Geometry: final body of the model. Coordinates: model frame, mm. A direction names the side the tool comes from. Give positions to 0.01 mm unless a question says otherwise; leave off trailing zeros. Order: outer loops, then holes, each group sorted by start corner. A loop starts at its lowest first (then second) coordinate and runs counter-clockwise, first axis right, second up. Notation, with made-up numbers: (85.25, -38.75) - (105.25, -38.75) arc R19 cw to (105.25, -21.75) - close; hole circle Ø7 at (2.5, -38). An arc over 180 degrees is marked (long way). One line per item, written item: value.
```python
from build123d import *

# Parameters (mm, degrees)
SKETCH1_R           = 1.651
SKETCH1_R_2         = 1.2446
BOSS_EXTRUDE1_DEPTH = 5.08
SKETCH2_R           = 5.40385
SKETCH2_R_2         = 4.1656
BOSS_EXTRUDE2_DEPTH = 1.0922
CHAMFER1_SIZE       = 0.889
SKETCH4_R           = 5.4102
SKETCH4_R_2         = 4.1656
BOSS_EXTRUDE3_DEPTH = 1.4986
CHAMFER2_SIZE       = 0.254


with BuildPart() as part:
    # Sketch1 → Boss-Extrude1 (new body)
    with BuildSketch(Plane(origin=(0, 0, 0), x_dir=(1, 0, 0), z_dir=(0, 1, 0))):
        with BuildLine():
            Line((-30.503852792, 3.086942476), (-1.192854484, 7.654613457))
            ThreePointArc((-1.192854484, 7.654613457), (0, 7.747), (1.192854484, 7.654613457))
            Line((1.192854484, 7.654613457), (30.503852792, 3.086942476))
            ThreePointArc((30.503852792, 3.086942476), (33.147, 0), (30.503852792, -3.086942476))
            Line((30.503852792, -3.086942476), (1.192854484, -7.654613457))
            ThreePointArc((1.192854484, -7.654613457), (0, -7.747), (-1.192854484, -7.654613457))
            Line((-1.192854484, -7.654613457), (-30.503852792, -3.086942476))
            ThreePointArc((-30.503852792, -3.086942476), (-33.147, 0), (-30.503852792, 3.086942476))
        make_face()
        Circle(SKETCH1_R, mode=Mode.SUBTRACT)
        with Locations((-10.0076, 0)):
            Circle(SKETCH1_R_2, mode=Mode.SUBTRACT)
        with Locations((-15.0114, 0)):
            Circle(SKETCH1_R_2, mode=Mode.SUBTRACT)
        with Locations((-20.0152, 0)):
            Circle(SKETCH1_R_2, mode=Mode.SUBTRACT)
        with Locations((-25.019, 0)):
            Circle(SKETCH1_R_2, mode=Mode.SUBTRACT)
        with Locations((-30.0228, 0)):
            Circle(SKETCH1_R_2, mode=Mode.SUBTRACT)
        with Locations((30.0228, 0)):
            Circle(SKETCH1_R_2, mode=Mode.SUBTRACT)
        with Locations((25.019, 0)):
            Circle(SKETCH1_R_2, mode=Mode.SUBTRACT)
        with Locations((20.0152, 0)):
            Circle(SKETCH1_R_2, mode=Mode.SUBTRACT)
        with Locations((15.0114, 0)):
            Circle(SKETCH1_R_2, mode=Mode.SUBTRACT)
        with Locations((10.0076, 0)):
            Circle(SKETCH1_R_2, mode=Mode.SUBTRACT)
    extrude(amount=BOSS_EXTRUDE1_DEPTH)

    # Sketch2 → Boss-Extrude2 (add)
    with BuildSketch(Plane(origin=(0, 5.08, 0), x_dir=(1, 0, 0), z_dir=(0, 1, 0))):
        Circle(SKETCH2_R)
        Circle(SKETCH2_R_2, mode=Mode.SUBTRACT)
    extrude(amount=BOSS_EXTRUDE2_DEPTH)

    # Chamfer1
    chamfer1_edges = [part.edges().sort_by_distance(p)[0] for p in [
        (-5.40385, 6.1722, 0),
    ]]
    chamfer(chamfer1_edges, length=CHAMFER1_SIZE)

    # Sketch4 → Boss-Extrude3 (add)
    with BuildSketch(Plane.XZ):
        Circle(SKETCH4_R)
        Circle(SKETCH4_R_2, mode=Mode.SUBTRACT)
    extrude(amount=BOSS_EXTRUDE3_DEPTH)

    # Chamfer2
    chamfer2_edges = [part.edges().sort_by_distance(p)[0] for p in [
        (-5.4102, -1.4986, 0),
    ]]
    chamfer(chamfer2_edges, length=CHAMFER2_SIZE)


solid = part.part
```
1) Material intervals for line 1 along Y through (x, z) = (-29, 1.25); line 2 along Z through (x, y) = (-25.5, 0.5); line 3 along Z through (x, y) = (9.5, 0.5), sorted ascending.
Answers below:
line 1: 0 to 5.08
line 2: -3.87 to -1.15, 1.15 to 3.87
line 3: -6.36 to -1.14, 1.14 to 6.36
2) Section C-C, the plane x = 14.5. Return loops of the section in (y, z).
Answers below:
outline: (0, -5.58) - (5.08, -5.58) - (5.08, -1.13) - (0, -1.13) - close; (0, 1.13) - (5.08, 1.13) - (5.08, 5.58) - (0, 5.58) - close
3) Section A-A, the plane x = 0. Return loops of the section in (y, z), then the cut area to 3 significant figures.
Answers below:
outline: (-1.5, -5.16) - (-1.24, -5.41) - (0, -5.41) - (0, -7.75) - (5.08, -7.75) - (5.08, -5.4) - (5.28, -5.4) - (6.17, -4.51) - (6.17, -4.17) - (5.08, -4.17) - (5.08, -1.65) - (0, -1.65) - (0, -4.17) - (-1.5, -4.17) - close; (-1.5, 4.17) - (0, 4.17) - (0, 1.65) - (5.08, 1.65) - (5.08, 4.17) - (6.17, 4.17) - (6.17, 4.51) - (5.28, 5.4) - (5.08, 5.4) - (5.08, 7.75) - (0, 7.75) - (0, 5.41) - (-1.24, 5.41) - (-1.5, 5.16) - close
area: 67.5 mm^2
4) Set-up query: faces 5 (the face through (-2, 5.08, 0)), 6 (the face through (3.973, -0.739, 1.251)), 7 (the face through (-11.25, 2.5, -0.05)). Return all of +Z, -Z, +X, -X, +Y, -Y with unobstructed straight access to the full face (end or side cutting, diameter ignored); none if empty.
Answers below:
face 5: +Y
face 6: -Y
face 7: +Y, -Y
5) Mould query, pull axis Z, two halves, no side actions, for faces 1 (the face through (0, 0, 7)), 2 (the face through (1.525, 2.504, 0.632)), 3 (the face through (16.05, 2.5, 5.34)), 4 (the face through (-21.26, 2.5, -0.05)). Classes: released by +Z, released by -Z, zero draft, split by the parting line, or undercut.
Answers below:
face 1: zero draft
face 2: undercut
face 3: released by +Z
face 4: undercut
6) Section B-B, the plane z = 0. Count the separate pieces of the cut face and the enclosed holes in it, then the cut area to 3 significant figures.
Answers below:
separate pieces: 12
enclosed holes: 0
area: 199 mm^2
7) Section D-D, the plane x = -17.5. Return loops of the section in (y, z), then the cut area to 3 significant figures.
Answers below:
outline: (0, -5.11) - (5.08, -5.11) - (5.08, 5.11) - (0, 5.11) - close
area: 52.0 mm^2
8) First-contact query: pin 1 (4 mm diameter, centred on x = 25.019, z = 0, fed in from +Y); pin 2 (1.5 mm diameter, centred on x = -1.5, y = 2.5, fed in from -Z); pin 3 (6 mm diameter, centred on x = 13, z = 1, fed in from -Y); pin 4 (2 mm diameter, centred on x = -25.019, z = 0, fed in from -Y). Flat tips, straight axial feed; report the tip coordinate or a pass-through.
Answers below:
pin 1: y = 5.08
pin 2: z = -7.71
pin 3: y = 0
pin 4: through
